The listing builds one solid part. Answer for the finished solid, in the listing's coordinates (mm). Round coordinates to 2 decimals unless told otherwise and drop trailing zeros. Order: outer loops, then holes, each group sorted by start corner. A loop starts at its lowest first (then second) coordinate and runs counter-clockwise, first axis right, second up. Notation, with made-up numbers: (25, -3) - (82, -3) arc R29 ccw to (82, 19) - close; hole circle Ø4 at (-35.5, 34.5). An arc over 180 degrees is marked (long way). Write item = value, one per line.
from build123d import *

# Parameters (mm, degrees)
PLAT_W                          = 50
PLAT_H                          = 5
EL_MENT_M_CANO_SOUD_1_DEPTH     = 70
DIAM_TRE_DU_PER_AGE_10_0_10_1_D = 10


with BuildPart() as part:
    # plat → Elément mécano-soudé1 (new body)
    with BuildSketch(Plane.YZ.offset(-35)):
        Rectangle(PLAT_W, PLAT_H)
    extrude(amount=EL_MENT_M_CANO_SOUD_1_DEPTH)

    # Diamètre du perçage Ø10.0 (10)1 (through all)
    with Locations(Plane(origin=(0, 0, -2.5), x_dir=(-1, 0, 0), z_dir=(0, 0, -1))):
        with Locations((20, 0)):
            Hole(DIAM_TRE_DU_PER_AGE_10_0_10_1_D / 2)


solid = part.part
Q1. Section A-A on y = 0 is taken. Determine the outline of the cut face in (x, z).
Model answer:
outline = (-35, -2.5) - (-25, -2.5) - (-25, 2.5) - (-35, 2.5) - close; (-15, -2.5) - (35, -2.5) - (35, 2.5) - (-15, 2.5) - close
Q2. Find the intervals of material crossed by line 1 (Y direction, x = -20, z = -0.75); line 2 (Y direction, x = -15.5, z = 0.9); line 3 (X direction, y = 1, z = 1.45), in increasing order. Write a range as from..to.
Model answer:
line_1 = -25..-5, 5..25
line_2 = -25..-2.18, 2.18..25
line_3 = -35..-24.9, -15.1..35
Q3. Determine the mould class of faces 1 (the face through (-35, 0, 0)), 2 (the face through (0, -25, 0)), 3 (the face through (0, 25, 0)), 4 (the face through (-25, 0, 0)) for opening direction Y: released by +Y, released by -Y, zero draft, split by the parting line, or undercut.
Model answer:
face_1 = zero draft
face_2 = released by -Y
face_3 = released by +Y
face_4 = undercut
Q4. Section B-B on x = -20 is taken. Determine the outline of the cut face in (y, z).
Model answer:
outline = (-25, -2.5) - (-5, -2.5) - (-5, 2.5) - (-25, 2.5) - close; (5, -2.5) - (25, -2.5) - (25, 2.5) - (5, 2.5) - close
Q5. Section C-C on z = 0.5 is taken. Determine the outline of the cut face in (x, y), then the cut area to 3 significant figures.
Model answer:
outline = (-35, -25) - (35, -25) - (35, 25) - (-35, 25) - close; hole circle Ø10 at (-20, 0)
area = 3,420 mm^2
